from build123d import *

# Parameters (mm, degrees)
SKETCH1_R           = 6.35
SKETCH1_R_2         = 12.7
BOSS_EXTRUDE1_DEPTH = 1.5875
FILLET1_R           = 25.4
FILLET2_R           = 25.4
FILLET3_R           = 25.4
FILLET4_R           = 25.4
FILLET5_R           = 12.7


with BuildPart() as part:
    # Sketch1 → Boss-Extrude1 (new body)
    with BuildSketch(Plane(origin=(0, 0, 0), x_dir=(0, 0, -1), z_dir=(1, 0, 0))):
        Polygon((-35.431920316, 38.1), (35.431920316, 38.1), (291.921947077, -30.626295537), (509.245567884, -407.04184846), (443.254432116, -445.14184846), (241.712348035, -96.060718969), (25.4, -38.1), (-25.4, -38.1), (-419.1, -143.59159706), (-419.1, -186.721280576), (-495.3, -186.721280576), (-495.3, -85.121280576), align=None)
        Circle(SKETCH1_R, mode=Mode.SUBTRACT)
        with Locations((457.2, -393.096280576)):
            Circle(SKETCH1_R_2, mode=Mode.SUBTRACT)
    extrude(amount=BOSS_EXTRUDE1_DEPTH)

    # Fillet1
    fillet1_edges = [part.edges().sort_by_distance(p)[0] for p in [
        (0.79375, -85.121280576, 495.3),
    ]]
    fillet(fillet1_edges, radius=FILLET1_R)

    # Fillet2
    fillet2_edges = [part.edges().sort_by_distance(p)[0] for p in [
        (0.79375, -143.59159706, 419.1),
    ]]
    fillet(fillet2_edges, radius=FILLET2_R)

    # Fillet3
    fillet3_edges = [part.edges().sort_by_distance(p)[0] for p in [
        (0.79375, -96.060718969, -241.712348035),
        (0.79375, -38.1, -25.4),
        (0.79375, -38.1, 25.4),
    ]]
    fillet(fillet3_edges, radius=FILLET3_R)

    # Fillet4
    fillet4_edges = [part.edges().sort_by_distance(p)[0] for p in [
        (0.79375, 38.1, 35.431920316),
        (0.79375, 38.1, -35.431920316),
        (0.79375, -30.626295537, -291.921947077),
    ]]
    fillet(fillet4_edges, radius=FILLET4_R)

    # Fillet5
    fillet5_edges = [part.edges().sort_by_distance(p)[0] for p in [
        (0.79375, -186.721280576, 419.1),
        (0.79375, -186.721280576, 495.3),
        (0.79375, -407.04184846, -509.245567884),
        (0.79375, -445.14184846, -443.254432116),
    ]]
    fillet(fillet5_edges, radius=FILLET5_R)


solid = part.part
Could you check a few things on this model? Use its own coordinates, in mm. A direction names the side the tool comes from. Coordinates: 2 decimals unless noted, no trailing zeros. Order: outer loops, then holes, each group sorted by start corner. A loop starts at its lowest first (then second) coordinate and runs counter-clockwise, first axis right, second up. Notation, with made-up numbers: (-4.75, 13.5) - (2.25, 13.5) arc R28 cw to (2.25, 48.5) - close; hole circle Ø3 at (78, 4). An arc over 180 degrees is marked (long way). Answer in a Markdown table with one row per item. Add a question column.
(1) If we section it at D-D, the plane z = 270: Please give me the cut outline in (x, y).
(2) Will these pins go through, and if not, where does the flat tip stop? pin 1 (0.5 mm diameter, centred on x = 1, z = 460, fed in from -Y); pin 2 (0.5 mm diameter, centred on x = 0.5, z = -10.5, fed in from -Y).
(3) I need wall thicknesses on L1, parallel to Y at x = 0.8, z = 0; L2, parallel to Y at x = 0.9, z = -16.5; L3, parallel to Y at x = 0.35, z = -449. Which ranges of each line are inside material? Lowest first, please.
(4) If we section it at A-A, the plane y = -57.5: Please give me the cut outline in (x, z).
(5) If we mould it in two halves opening along Z, with no side actions, what happens to faces 1 (the face through (0.805, -88.965, 489.909)), 2 (the face through (1.588, -41, -44)), 3 (the face through (0.783, -66.532, -131.51))? For each: released by +Z, released by -Z, zero draft, split by the parting line, or undercut.
(6) If we section it at C-C, the plane y = -199: Please give me the cut outline in (x, z), then the cut area to 3 significant figures.
(7) If we section it at B-B, the plane x = 0.7: Please give me the cut outline in (y, z), then the cut area to 3 significant figures.
(8) On a 3-axis mill with a long thin cutter (end or side, diameter ignored), from which of +Z, -Z, +X, -X, +Y, -Y can I reach the whole of each face in a straight line? I mean faces 4 (the face through (0.78, -271.96, -343.27)), 5 (the face through (0.783, -404.363, -463.06)). Say none if no direction works.
Results are:
| question | item | result |
|---|---|---|
| 1 | outline | (0, -103.64) - (1.59, -103.64) - (1.59, -24.75) - (0, -24.75) - close |
| 2 | pin 1 | stops at y = -186.72 |
| 2 | pin 2 | stops at y = -38.1 |
| 3 | L1 | y = -38.1 to -6.35, 6.35 to 38.1 |
| 3 | L2 | y = -38.1 to 38.1 |
| 3 | L3 | y = -440.45 to -402.79, -383.4 to -302.69 |
| 4 | outline | (0, -307.44) - (1.59, -307.44) - (1.59, -97.8) - (0, -97.8) - close; (0, 97.8) - (1.59, 97.8) - (1.59, 392.22) - (0, 392.22) - close |
| 5 | face 1 | released by +Z |
| 5 | face 2 | zero draft |
| 5 | face 3 | undercut |
| 6 | outline | (0, -389.13) - (1.59, -389.13) - (1.59, -301.14) - (0, -301.14) - close |
| 6 | area | 140 mm2 |
| 7 | outline | (-438.79, -454.25) - (-413.39, -498.25) arc R12.7 ccw to (-396.04, -502.9) - (-39.74, -297.18) arc R25.4 ccw to (-27.9, -281.76) - (37.23, -38.66) arc R25.4 ccw to (38.1, -32.09) - (38.1, 32.09) arc R25.4 ccw to (37.23, 38.66) - (-80.08, 476.47) arc R25.4 ccw to (-104.61, 495.3) - (-174.02, 495.3) arc R12.7 ccw to (-186.72, 482.6) - (-186.72, 431.8) arc R12.7 ccw to (-174.02, 419.1) - (-163.08, 419.1) arc R25.4 cw to (-138.55, 400.27) - (-38.97, 28.63) arc R25.4 cw to (-38.1, 22.06) - (-38.1, -22.06) arc R25.4 cw to (-38.97, -28.63) - (-93.34, -231.55) arc R25.4 cw to (-105.17, -246.97) - (-434.14, -436.9) arc R12.7 ccw to start; hole circle Ø25.4 at (-393.1, -457.2); hole circle Ø12.7 at (0, 0) |
| 7 | area | 93,600 mm2 |
| 8 | face 4 | +X, -X, -Y |
| 8 | face 5 | +X, -X |
